Part model, mm, in its own coordinate system. Give positions to 0.01 mm unless a question says otherwise; leave off trailing zeros. Write each loop counter-clockwise with the first axis right and the second up, starting at its lowest first coordinate (ties: lowest second). Pieces come first, ordered by that corner, then holes. Notation, with made-up numbers: M 32,81 L 54,81 A22 ccw 54,101 Z; hole C 27,81.5 d11. An arc over 180 degrees is marked long. Use a Markdown table: item, result.
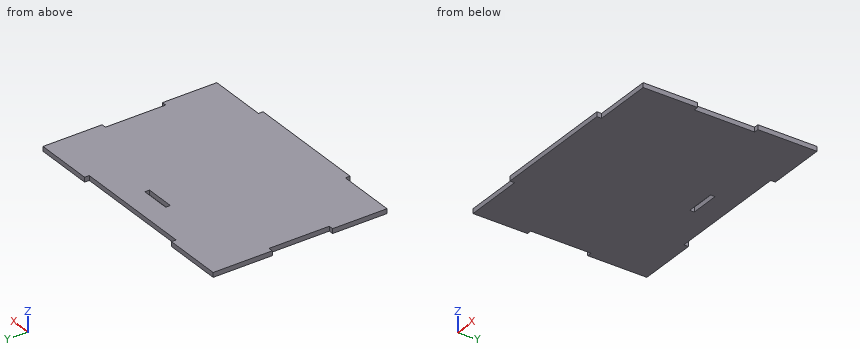
```python
from build123d import *

# Parameters (mm, degrees)
SKETCH1_W           = 12.7
SKETCH1_H           = 2
BOSS_EXTRUDE1_DEPTH = 2


with BuildPart() as part:
    # Sketch1 → Boss-Extrude1 (new body)
    with BuildSketch(Plane.XY):
        Polygon((-26.543, 36.354), (26.543, 36.354), (26.543, 38.354), (51.943, 38.354), (51.943, 12.954), (49.943, 12.954), (49.943, -12.954), (51.943, -12.954), (51.943, -36.354), (49.943, -36.354), (26.543, -36.354), (26.543, -38.354), (-26.543, -38.354), (-26.543, -36.354), (-49.943, -36.354), (-51.943, -36.354), (-51.943, -12.954), (-49.943, -12.954), (-49.943, 12.954), (-51.943, 12.954), (-51.943, 38.354), (-26.543, 38.354), align=None)
        with Locations((0, 25.654)):
            Rectangle(SKETCH1_W, SKETCH1_H, mode=Mode.SUBTRACT)
    extrude(amount=BOSS_EXTRUDE1_DEPTH)


solid = part.part
```
1. Cut at A-A, the plane z = 1.2. Give the cut face in (x, y).
Findings below:
| item | result |
|---|---|
| outline | M -51.94,-36.35 L -26.54,-36.35 L -26.54,-38.35 L 26.54,-38.35 L 26.54,-36.35 L 51.94,-36.35 L 51.94,-12.95 L 49.94,-12.95 L 49.94,12.95 L 51.94,12.95 L 51.94,38.35 L 26.54,38.35 L 26.54,36.35 L -26.54,36.35 L -26.54,38.35 L -51.94,38.35 L -51.94,12.95 L -49.94,12.95 L -49.94,-12.95 L -51.94,-12.95 Z; hole M -6.35,24.65 L 6.35,24.65 L 6.35,26.65 L -6.35,26.65 Z |
2. Cut at C-C, the plane x = -28.5. Give the cut face in (y, z).
Findings below:
| item | result |
|---|---|
| outline | M -36.35,0 L 38.35,0 L 38.35,2 L -36.35,2 Z |
3. Cut at B-B, the plane y = -9. Give the cut face in (x, z).
Findings below:
| item | result |
|---|---|
| outline | M -49.94,0 L 49.94,0 L 49.94,2 L -49.94,2 Z |
4. Drop flat-ended pins along their axis: P1, Ø1, axis at x = -37, z = 1, coming from the -Y side; P2, Ø0.6, axis at x = 1.5, z = 0.5, coming from the +Y side; P3, Ø0.6, axis at y = -0.5, z = 1, coming from the -X side. Give the stop position or say it passes through.
Findings below:
| item | result |
|---|---|
| P1 | y = -36.35 |
| P2 | y = 36.35 |
| P3 | x = -49.94 |
5. Drill centre lines: L1, parallel to Y at x = -5, z = 1.3; L2, parallel to Y at x = 22.5, z = 1.8; L3, parallel to Y at x = 44, z = 0.2. Where is each one in solid material? Low to high.
Findings below:
| item | result |
|---|---|
| L1 | -38.35 to 24.65, 26.65 to 36.35 |
| L2 | -38.35 to 36.35 |
| L3 | -36.35 to 38.35 |
